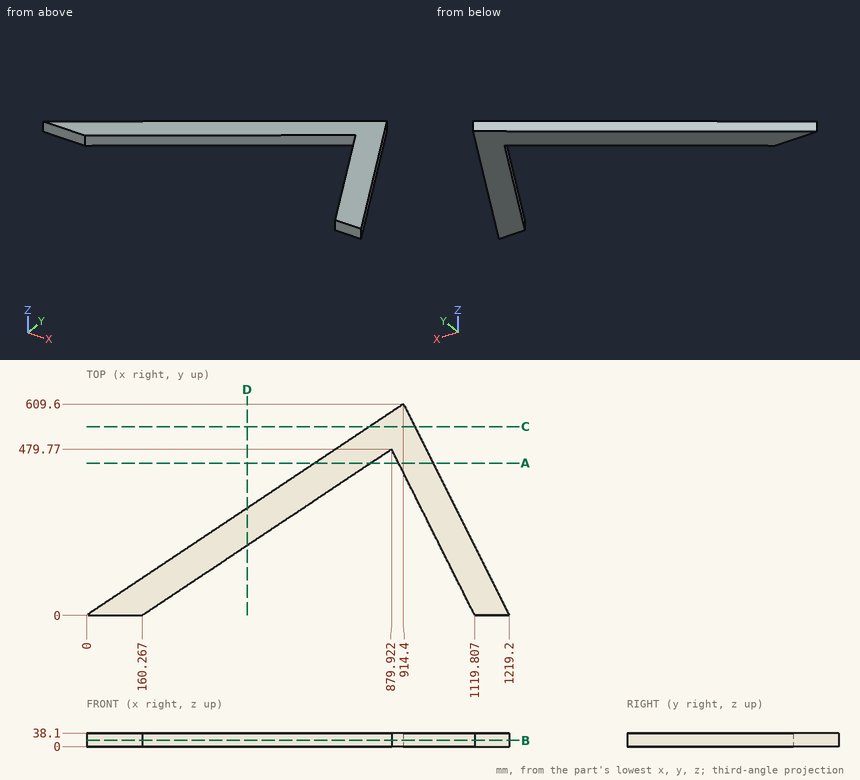
Answer from the drawing. Dimensions are ordinates in mm from the lowest x, y and z of the part. Round coordinates to 2 decimals unless told otherwise and drop trailing zeros. Loops run counter-clockwise (first coordinate to the right, second up) from the corner with the lowest first, then second, coordinate; pieces in that order, holes last. Notation, with made-up numbers: M -30.5,51.5 L 9.5,51.5 A34 cw 9.5,89.5 Z; hole C 14,-7 d1. An arc over 180 degrees is marked long. One line per question, with ' | ' between items. Start each with the question number.
(1) A cutting plane is placed at D-D on x = 463.5. Write down the section's boundary in (y, z).
(2) A cutting plane is placed at C-C on y = 544. Write down the section's boundary in (x, z).
(3) Find the intervals of material crossed by line 1 (X direction, y = 372.5, z = 15); line 2 (X direction, y = 423.5, z = 2); line 3 (Y direction, x = 648.5, z = 21), in increasing order.
(4) Flat-ended cylindrical pins translate along their axes: pin 1 Ø1 at (x, z) = (253, 18.5) entering from -Y; pin 2 Ø8 at (x, z) = (753, 20.5) entering from +Y; pin 3 Ø12 at (y, z) = (405.5, 22) entering from +X. Find the tip coordinate at first contact, or state that the pin passes through.
(5) A cutting plane is placed at B-B on z = 18. Write down the section's boundary in (x, y).
(6) A cutting plane is placed at A-A on y = 439. Write down the section's boundary in (x, z), plus the area to 3 significant figures.
Geometry check:
1) outline: M 202.16,0 L 309,0 L 309,38.1 L 202.16,38.1 Z
2) outline: M 816,0 L 947.2,0 L 947.2,38.1 L 816,38.1 Z
3) line 1: x = 558.75 to 719.02, 933.56 to 1032.95 | line 2: x = 635.25 to 795.52, 908.06 to 1007.45 | line 3: y = 325.49 to 432.33
4) pin 1: stops at y = 61.49 | pin 2: stops at y = 504.67 | pin 3: stops at x = 1019.45
5) outline: M 0,0 L 160.27,0 L 879.92,479.77 L 1119.81,0 L 1219.2,0 L 914.4,609.6 Z
6) outline: M 658.5,0 L 818.77,0 L 818.77,38.1 L 658.5,38.1 Z; M 900.31,0 L 999.7,0 L 999.7,38.1 L 900.31,38.1 Z | area: 9,890 mm²
